```python
from build123d import *

# Parameters (mm, degrees)
F0_W     = 25.4
F0_H     = 25.4
F1_DEPTH = 444.5
F2_W     = 25.4
F2_H     = 25.4
F3_DEPTH = 209.55
F5_W     = 25.4
F5_H     = 25.4
F6_DEPTH = 50.8
F7_R     = 1.5875
F8_DEPTH = 25.4


with BuildPart() as f1:
    # F0 (on Top) → F1 (new body)
    with BuildSketch(Plane.XY):
        with Locations((-222.25, 0)):
            Rectangle(F0_W, F0_H)
    extrude(amount=F1_DEPTH)

    # F2 (on face) → F3 (join)
    with BuildSketch(Plane.YZ.offset(-209.55)):
        with Locations((0, 431.8)):
            Rectangle(F2_W, F2_H)
    extrude(amount=F3_DEPTH)

    # F4: F1 across plane


with BuildPart() as f1_1:
    add(f1.part)
    add(f1.part.mirror(Plane.YZ))

    # F5 (on face) → F6 (join)
    with BuildSketch(Plane(origin=(0, 0, 419.1), x_dir=(1, 0, 0), z_dir=(0, 0, -1))):
        Rectangle(F5_W, F5_H)
    extrude(amount=F6_DEPTH)

    # F7 (on face) → F8 (join)
    with BuildSketch(Plane.XZ.offset(12.7)):
        with Locations((0, 381)):
            Circle(F7_R)
    extrude(amount=F8_DEPTH)


solid = f1_1.part
```
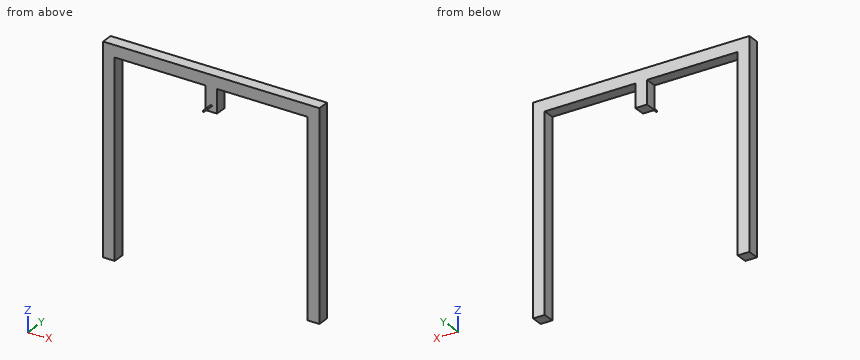
For this review, take the finished solid that the model builds, in its own axes (mm). Coordinates: 2 decimals unless noted, no trailing zeros. Loops run counter-clockwise (first coordinate to the right, second up) from the corner with the lowest first, then second, coordinate; pieces in that order, holes last. Notation, with made-up numbers: (-4.5, 61) -> (6.5, 61) arc R7 cw to (6.5, 67) -> close; hole circle Ø2 at (-36.5, 7.25). An arc over 180 degrees is marked (long way). Return JSON: item names as keys, results as strings. Group by question number.
(1) Consider section A-A, the plane z = 352. Give the boundary of the cut face in (x, y), plus the area to 3 significant figures.
(2) Consider section C-C, the plane x = -159.5. Give the boundary of the cut face in (y, z), plus the area to 3 significant figures.
(3) Consider section B-B, the plane y = -25.5. Give the boundary of the cut face in (x, z) (1 decimal), plus the area to 3 significant figures.
(4) For pin 1 Ø20.5 at (x, y) = (-3, -1.5) entering from -Z; pin 2 Ø7.5 at (x, y) = (-141.5, -1.5) entering from -Z, all flat-tipped, find the tip position at first contact; note any pin that passes through.
(5) To check wall thickness, follow L1, parallel to X at y = -12, z = 236.5; L2, parallel to Z at x = 153, y = -11.5. State the ranges of each line that lie inside material, in increasing order.
Results below:
{
 "1": {"outline": "(-234.95, -12.7) -> (-209.55, -12.7) -> (-209.55, 12.7) -> (-234.95, 12.7) -> close; (209.55, -12.7) -> (234.95, -12.7) -> (234.95, 12.7) -> (209.55, 12.7) -> close", "area": "1,290 mm2"},
 "2": {"outline": "(-12.7, 419.1) -> (12.7, 419.1) -> (12.7, 444.5) -> (-12.7, 444.5) -> close", "area": "645 mm2"},
 "3": {"outline": "circle Ø3.2 at (0, 381)", "area": "7.92 mm2"},
 "4": {"pin 1": "stops at z = 368.3", "pin 2": "stops at z = 419.1"},
 "5": {"L1": "x = -234.95 to -209.55, 209.55 to 234.95", "L2": "z = 419.1 to 444.5"}
}
